Autodesk Fusion 360 part; units mm, degrees
sketch "Esquisse1" plane through (0, 0, 0) normal (0, 0, 1) x (1, 0, 0)
  line L0 (17, 0) -> (0, 0)
  line L1 (0, 0) -> (0, 72)
  line L2 (0, 72) -> (17, 72)
  line L3 (17, 72) -> (17, 0)
  dimension "d3" = 72
  dimension "d4" = 17
extrude "Extrusion1" add sketch "Esquisse1" along normal blind 9
sketch "Esquisse2" plane through (0, 0, 0) normal (0, -1, 0) x (1, 0, 0)
  line L0 (0, 0) -> (17, 0)
  line L1 (17, 9) -> (0, 9)
  line L2 (0, 9) -> (0, 0)
  line L3 (-5.7525, 4.5) -> (21.5406, 4.5) construction
  circle A0 centre (5, 4.5) radius 2.175
  circle A1 centre (12, 4.5) radius 2.175
  line L4 (17, 0) -> (17, 9)
  dimension "d7" = 4.35
  dimension "d8" = 7
  dimension "d9" = 4.5
  dimension "d10" = 5
extrude "Extrusion2" cut sketch "Esquisse2" against normal blind 8 contours A0 | A1
sketch "Esquisse3" plane through (0, 72, 0) normal (0, 1, 0) x (-1, 0, 0)
  line L0 (-17, 0) -> (0, 0)
  line L1 (0, 0) -> (0, 9)
  line L2 (0, 9) -> (-17, 9)
  line L3 (5.6122, 4.5) -> (-27.7174, 4.5) construction
  circle A0 centre (-12, 4.5) radius 2.175
  circle A1 centre (-5, 4.5) radius 2.175
  line L4 (-17, 9) -> (-17, 0)
  dimension "d13" = 4.5
  dimension "d14" = 7
  dimension "d15" = 5
  dimension "d16" = 4.35
extrude "Extrusion3" cut sketch "Esquisse3" against normal blind 8 contours A0 | A1
sketch "Esquisse9" plane through (0, 0, 0) normal (-1, 0, 0) x (0, 0, 1)
  line L0 (0, 72) -> (0, 0)
  line L1 (0, 0) -> (9, 0)
  line L2 (9, 0) -> (9, 72)
  line L3 (9, 72) -> (0, 72)
  line L4 (9, 65) -> (-15, 65)
  line L5 (-15, 65) -> (-15, 48.5)
  line L6 (-15, 48.5) -> (9, 48.5)
  line L7 (9, 48.5) -> (9, 65)
  line L8 (9, 7) -> (-15, 7)
  line L9 (-15, 7) -> (-15, 23.5)
  line L10 (-15, 23.5) -> (9, 23.5)
  line L11 (9, 23.5) -> (9, 7)
  line L12 (6.675, 72) -> (2.325, 72)
  dimension "d48" = 7
  dimension "d49" = 7
  dimension "d50" = 25
  dimension "d51" = 15
extrude "Extrusion7" add sketch "Esquisse9" against normal blind 10 contours L0 L4 L5 L6 | L0 L8 L9 L10
sketch "Esquisse10" plane through (0, 7, 0) normal (0, -1, 0) x (1, 0, 0)
  line L0 (0, -15) -> (10, -15)
  line L1 (10, -15) -> (10, 0)
  line L2 (10, 0) -> (0, 0)
  line L3 (0, 0) -> (0, -15)
  circle A0 centre (5, -10) radius 2.175
  dimension "d56" = 4.35
  dimension "d57" = 5
  dimension "d76" = 5
extrude "Extrusion9" cut sketch "Esquisse10" against normal blind 61 contours A0
sketch "Esquisse11" plane through (0, 48.5, 0) normal (0, -1, 0) x (1, 0, 0)
  circle A0 centre (5, -10) radius 2.175
  line L0 (10, -15) -> (10, 0)
  line L1 (10, 0) -> (0, 0)
  line L2 (0, 0) -> (0, -15)
  line L3 (0, -15) -> (10, -15)
chamfer "Chanfrein4" distance 7 distance2 3 1 edges at (17, 36, 0) measured on face at (3.3333, 40.1667, 0)
sketch "Esquisse12" plane through (0, 0, -15) normal (0, 0, -1) x (-1, 0, 0)
  line L0 (0, 48.5) -> (0, 65)
  line L1 (0, 65) -> (-10, 65)
  line L2 (-10, 65) -> (-10, 48.5)
  line L3 (-10, 48.5) -> (0, 48.5)
  line L4 (-10, 65) -> (0, 65)
  line L5 (0, 65) -> (0, 7)
  line L6 (0, 7) -> (-10, 7)
  line L7 (-10, 7) -> (-10, 65)
  line L8 (0, 7) -> (-10, 7)
extrude "Extrusion10" add sketch "Esquisse12" along normal blind 10
extrude "Extrusion11" add 1 faces at (3.3333, 31.8333, -15) along direction (0, 0, 1) up to surface (15 mm away)
sketch "Esquisse13" plane through (0, 0, -25) normal (0, 0, -1) x (-1, 0, 0)
  line L0 (0, 7) -> (0, 65)
  line L1 (-10, 65) -> (-10, 7)
  line L2 (-10, 27) -> (-17, 27)
  line L3 (-17, 27) -> (-17, 45)
  line L4 (-17, 45) -> (-10, 45)
  line L5 (-10, 45) -> (-10, 27)
  line L6 (0, 65) -> (-10, 65)
  line L7 (-10, 7) -> (0, 7)
  dimension "d82" = 7
extrude "Extrusion12" add sketch "Esquisse13" against normal blind 28 contours L1 L2 L3 L4 L5
sketch "Esquisse15" plane through (17, 0, 0) normal (1, 0, 0) x (0, 0, -1)
  line L0 (-3, 45) -> (-3, 72)
  line L1 (-3, 72) -> (-9, 72)
  line L2 (-9, 72) -> (-9, 0)
  line L3 (-9, 0) -> (-3, 0)
  line L4 (16.5, 30.5) -> (-2, 30.5)
  line L5 (-2, 30.5) -> (-2, 41.5)
  line L6 (-2, 41.5) -> (16.5, 41.5)
  line L7 (16.5, 41.5) -> (16.5, 30.5)
  line L8 (-3, 0) -> (-3, 27)
  line L9 (-3, 27) -> (25, 27)
  line L10 (25, 27) -> (25, 45)
  line L11 (25, 45) -> (-3, 45)
  dimension "d96" = 7
extrude "Extrusion13" cut sketch "Esquisse15" against normal blind 27 contours L4 L5 L6 L7
chamfer "Chanfrein6" distance 3 angle 45 6 edges at (17, 27, -11) (17, 45, -11) (13.5, 27, -25) (13.5, 45, -25) (0, 41.5, -7.25) (0, 30.5, -7.25)
chamfer "Chanfrein7" distance 5 distance2 5 2 edges at (10, 53.5, -25) (10, 18.5, -25) measured on face at (3.3333, 38, -25) measured on face at (3.3333, 38, -25)
chamfer "Chanfrein8" distance 10 distance2 10 2 edges at (2.5, 65, -25) (2.5, 7, -25) measured on face at (13, 38, -25) measured on face at (13, 38, -25)
equation "d49 = d48"
Input: part model. Units: mm. Frame: model coordinates. A direction names the side the tool comes from. Coordinates: 2 decimals unless noted, no trailing zeros. Order: outer loops, then holes, each group sorted by start corner. A loop starts at its lowest first (then second) coordinate and runs counter-clockwise, first axis right, second up. Notation, with made-up numbers: (42, 47.5) - (76, 47.5) arc R32 ccw to (76, 75.5) - close; hole circle Ø4 at (51, 67). An arc over 180 degrees is marked (long way). Put each result on its own line as item: value.
1. Draft query along X for faces 4 (the face through (6, 56.63, -11.93)), 5 (the face through (0, 27, -8)), 6 (the face through (13.5, 57.2, 1.5)). Return one class per face: pulls with the +X half, pulls with the -X half, needs draft (parallel to the pull), parting line crosses it, or undercut.
Report:
face 4: undercut
face 5: pulls with the -X half
face 6: pulls with the +X half
2. Cut plane C-C on z = -19. Return the cut outline in (x, y), then the cut area to 3 significant figures.
Report:
outline: (0, 11) - (10, 11) - (10, 27) - (14, 27) - (17, 30) - (17, 42) - (14, 45) - (10, 45) - (10, 61) - (0, 61) - close
area: 617 mm2
3. Cut plane A-A on z = -2. Return the cut outline in (x, y), then the cut area to 3 significant figures.
Report:
outline: (0, 7) - (10, 7) - (10, 27) - (14, 27) - (17, 30) - (17, 30.5) - (3, 30.5) - (0, 27.5) - close; (0, 44.5) - (3, 41.5) - (17, 41.5) - (17, 42) - (14, 45) - (10, 45) - (10, 65) - (0, 65) - close
area: 501 mm2
4. Line query: line 1 along Z through (x, y) = (5, 67) (3 decimals); line 2 along Y through (x, z) = (7.75, 1.5); line 3 along Y through (x, z) = (14, -11.5). Output: solid intervals per line, ascending.
Report:
line 1: z = 0 to 2.325, 6.675 to 9
line 2: y = 0 to 30.5, 41.5 to 72
line 3: y = 27 to 30.5, 41.5 to 45
5. Reachability of faces 1 (the face through (16, 29, -11)), 2 (the face through (1.5, 43, -7.1)), 3 (the face through (5, 7, -7)) from +Z, -Z, +X, -X, +Y, -Y: full face, straight path, thin tool, end or side. Return the list, or none.
Report:
face 1: -Z, +X, -Y
face 2: -X
face 3: -Z, +X, -X, -Y
6. Contact query for flat-ended pins moving along their axis: pin 1 Ø3.5 at (x, z) = (5, 4.5) entering from +Y; pin 2 Ø5 at (x, y) = (4, 64) entering from -Z; pin 3 Ø1.5 at (x, z) = (10, -2) entering from -Y. Output: stop coordinate, or through.
Report:
pin 1: stops at y = 64
pin 2: stops at z = -18.5
pin 3: stops at y = 7
7. Cut plane D-D on x = 12. Return the cut outline in (y, z) (3 decimals), then the cut area to 3 significant figures.
Report:
outline: (0, 0.857) - (27, 0.857) - (27, -22) - (30, -25) - (42, -25) - (45, -22) - (45, 0.857) - (72, 0.857) - (72, 2.325) - (64, 2.325) - (64, 6.675) - (72, 6.675) - (72, 9) - (0, 9) - (0, 6.675) - (8, 6.675) - (8, 2.325) - (0, 2.325) - close; hole (30.5, -16.5) - (41.5, -16.5) - (41.5, 2) - (30.5, 2) - close
area: 770 mm2
